from build123d import *

# Parameters (mm, degrees)
F1_DEPTH = 6.35
F2_R     = 6.35
F3_DEPTH = 127
F4_SIZE  = 1.27


with BuildPart() as f1:
    # F0 (on Front) → F1 (new body)
    with BuildSketch(Plane.XZ):
        Polygon((6.351873, -11.149167), (12.831398, -0.0737), (6.479525, 11.075467), (-6.351873, 11.149167), (-12.831398, 0.0737), (-6.479525, -11.075467), align=None)
    extrude(amount=F1_DEPTH)

    # F2 (on Front) → F3 (join)
    with BuildSketch(Plane.XZ):
        Circle(F2_R)
    extrude(amount=F3_DEPTH)

    # F4
    f4_edges = [f1.edges().sort_by_distance(p)[0] for p in [
        (-6.35, -127, 0),
    ]]
    chamfer(f4_edges, length=F4_SIZE)


solid = f1.part
Geometry check sheet. Reference: the model listing, model coordinates, mm. A direction names the side the tool comes from. Round coordinates to 2 decimals unless told otherwise and drop trailing zeros. Order: outer loops, then holes, each group sorted by start corner. A loop starts at its lowest first (then second) coordinate and runs counter-clockwise, first axis right, second up. Notation, with made-up numbers: (-8, 77) - (44, 77) arc R17 cw to (44, 106) - close; hole circle Ø5 at (74, -28.75). An arc over 180 degrees is marked (long way). One line per question, with ' | ' between items. Start each with the question number.
(1) Thickness scan on L1, parallel to Y at x = 5.5, z = 5.75; L2, parallel to X at y = -99, z = 4; L3, parallel to Z at x = -2, y = -84. Record the ranges inside material, lowest first. Write a range as [from, to].
(2) Sectioned sample at D-D on x = 8.75. Record the cut outline in (y, z), and give its area (3 significant figures).
(3) Sectioned sample at B-B on y = -114. Record the cut outline in (x, z), and give its area (3 significant figures).
(4) Sectioned sample at C-C on z = 9.5. Record the cut outline in (x, y).
(5) Depth check by flat-ended pin: pin 1 Ø8 at (x, y) = (-1.5, -74) entering from +Z; pin 2 Ø12 at (y, z) = (-68.5, 8) entering from -X; pin 3 Ø1 at (y, z) = (-100, 8) entering from +X; pin 4 Ø1.5 at (x, z) = (8, -4.5) entering from -Y. Enter the tip coordinate at first touch or a pass-through.
(6) Access from +Z, -Z, +X, -X, +Y, -Y to the whole of each face (thin tool, end or side, straight path). Record for faces 1 (the flat face through (9.546, -3.131, -5.689)), 2 (the cylindrical face through (-1.38, -65.2, -6.2)).
(7) Sectioned sample at A-A on x = 0. Record the cut outline in (y, z), and give its area (3 significant figures).
Conclusion:
1) L1: y = [-6.35, 0] | L2: x = [-4.93, 4.93] | L3: z = [-6.03, 6.03]
2) outline: (-6.35, -7.05) - (0, -7.05) - (0, 7.09) - (-6.35, 7.09) - close | area: 89.8 mm2
3) outline: circle Ø12.7 at (0, 0) | area: 127 mm2
4) outline: (-7.32, -6.35) - (7.38, -6.35) - (7.38, 0) - (-7.32, 0) - close
5) pin 1: stops at z = 6.35 | pin 2: stops at x = -6.03 | pin 3: passes through | pin 4: stops at y = -6.35
6) face 1: -Z, +X, +Y, -Y | face 2: -Y
7) outline: (-127, -5.08) - (-125.73, -6.35) - (-6.35, -6.35) - (-6.35, -11.11) - (0, -11.11) - (0, 11.11) - (-6.35, 11.11) - (-6.35, 6.35) - (-125.73, 6.35) - (-127, 5.08) - close | area: 1,670 mm2
